```python
from build123d import *

# Parameters (mm, degrees)
F0_R           = 20
F1_DEPTH       = 2
F3_D           = 3.5
F3_CBORE_D     = 5.5
F3_CBORE_DEPTH = 3
F4_D           = 16


with BuildPart() as f1:
    # F0 (on Front) → F1 (new body, symmetric)
    with BuildSketch(Plane.XZ):
        Circle(F0_R)
    extrude(amount=F1_DEPTH, both=True)

    # F3 (through all)
    with Locations(Plane.XZ.offset(2)):
        with Locations((0, 15), (-15, 0), (0, -15), (15, 0)):
            CounterBoreHole(F3_D / 2, F3_CBORE_D / 2, F3_CBORE_DEPTH)

    # F4 (through all)
    with Locations(Plane.XZ.offset(2)):
        with Locations((0, 0)):
            Hole(F4_D / 2)


solid = f1.part
```
Verification items for the finished model (mm, model axes). A direction names the side the tool comes from. Round coordinates to 2 decimals unless told otherwise and drop trailing zeros. Write each loop counter-clockwise with the first axis right and the second up, starting at its lowest first coordinate (ties: lowest second). Pieces come first, ordered by that corner, then holes.
1. Gauge pin test, flat ends, axial feed: P1, Ø4, axis at x = 15, z = 0, coming from the -Y side; P2, Ø9, axis at x = -15, z = 0, coming from the -Y side; P3, Ø1, axis at y = -1.5, z = -9.5, coming from the +X side; P4, Ø2, axis at x = -12, y = 0.5, coming from the -Z side. Record the tip position at first contact, or that the pin passes through.
2. Draft check along Z on faces 3 (the cylindrical face through (-4.336, -0.028, -19.524)), 4 (the flat face through (9, -2, 0)), 5 (the cylindrical face through (-0.358, -0.521, -12.273)). Enter one of: +Z half, -Z half, draft (parallel to the pull), parting line (faces both ways), or undercut.
3. Access from +Z, -Z, +X, -X, +Y, -Y to the whole of each face (thin tool, end or side, straight path). Record for faces 1 (the cylindrical face through (0.228, 1.507, 16.735)), 2 (the flat face through (15, 1, -2)).
4. Section check A-A on z = 0. Enter the section's corners in (x, y), plus the area to 3 significant figures.
5. Section check B-B on x = 0. Enter the section's corners in (y, z).
6. Section check C-C on y = 0.5. Enter the section's corners in (x, z).
7. Section check D-D on x = -14. Enter the section's corners in (y, z), plus the area to 3 significant figures.
8. Scan lines: L1, parallel to Z at x = 0, y = 1.55; L2, parallel to Z at x = 0, y = -0.1; L3, parallel to X at y = -1.7, z = -4. Record each from-to range of solid material in increasing order.
Answer:
1. P1: stops at y = 1
1. P2: stops at y = -2
1. P3: stops at x = 17.86
1. P4: stops at z = -16.7
2. face 3: parting line
2. face 4: draft
2. face 5: undercut
3. face 1: +Y, -Y
3. face 2: -Y
4. outline: (-20, -2) - (-17.75, -2) - (-17.75, 1) - (-16.75, 1) - (-16.75, 2) - (-20, 2) - close; (-13.25, 1) - (-12.25, 1) - (-12.25, -2) - (-8, -2) - (-8, 2) - (-13.25, 2) - close; (8, -2) - (12.25, -2) - (12.25, 1) - (13.25, 1) - (13.25, 2) - (8, 2) - close; (16.75, 1) - (17.75, 1) - (17.75, -2) - (20, -2) - (20, 2) - (16.75, 2) - close
4. area: 56.0 mm2
5. outline: (-2, -20) - (2, -20) - (2, -16.75) - (1, -16.75) - (1, -17.75) - (-2, -17.75) - close; (-2, -12.25) - (1, -12.25) - (1, -13.25) - (2, -13.25) - (2, -8) - (-2, -8) - close; (-2, 8) - (2, 8) - (2, 13.25) - (1, 13.25) - (1, 12.25) - (-2, 12.25) - close; (-2, 17.75) - (1, 17.75) - (1, 16.75) - (2, 16.75) - (2, 20) - (-2, 20) - close
6. outline: circle Ø40 at (0, 0); hole circle Ø5.5 at (-15, 0); hole circle Ø16 at (0, 0); hole circle Ø5.5 at (0, -15); hole circle Ø5.5 at (0, 15); hole circle Ø5.5 at (15, 0)
7. outline: (-2, -14.28) - (2, -14.28) - (2, -1.44) - (1, -1.44) - (1, -2.56) - (-2, -2.56) - close; (-2, 2.56) - (1, 2.56) - (1, 1.44) - (2, 1.44) - (2, 14.28) - (-2, 14.28) - close
7. area: 96.0 mm2
8. L1: z = -20 to -16.75, -13.25 to -8, 8 to 13.25, 16.75 to 20
8. L2: z = -20 to -17.75, -12.25 to -8, 8 to 12.25, 17.75 to 20
8. L3: x = -19.6 to -6.93, 6.93 to 19.6
